```python
from build123d import *

# Parameters (mm, degrees)
SALIENTE_EXTRUIR1_DEPTH = 15.875
REDONDEO1_R             = 15.875
CORTAR_EXTRUIR1_REACH   = 48.084
CROQUIS2_R              = 9.525
CORTAR_EXTRUIR2_START   = -3.175
CROQUIS3_R              = 12.7
CORTAR_EXTRUIR2_DEPTH   = 43.909243503
CROQUIS4_R              = 3.2639
CROQUIS4_R_2            = 2.4892
CORTAR_EXTRUIR3_DEPTH   = 47.084243503
REDONDEO2_R             = 1.27
REDONDEO3_R             = 2.54


with BuildPart() as part:
    # Croquis1 → Saliente-Extruir1 (new body)
    with BuildSketch(Plane.XY):
        Polygon((30.48, 0), (-30.48, 0), (-30.48, 6.35), (12.046472996, 38.277805334), (30.48, 6.35), align=None)
    extrude(amount=SALIENTE_EXTRUIR1_DEPTH)

    # Redondeo1
    redondeo1_edges = [part.edges().sort_by_distance(p)[0] for p in [
        (12.046472996, 38.277805334, 7.9375),
    ]]
    fillet(redondeo1_edges, radius=REDONDEO1_R)

    # Croquis2 → Cortar-Extruir1 (cut, up to next)
    with BuildSketch(Plane.XY.offset(15.875), mode=Mode.PRIVATE) as cortar_extruir1_sk1:
        with Locations((7.254003, 16.09860686)):
            Circle(CROQUIS2_R)
    cortar_extruir1_tool1 = extrude(cortar_extruir1_sk1.sketch, amount=-CORTAR_EXTRUIR1_REACH, mode=Mode.PRIVATE) & part.part
    add(cortar_extruir1_tool1.solids().sort_by_distance((7.254003, 16.098607, 15.875))[0], mode=Mode.SUBTRACT)

    # Croquis3 → Cortar-Extruir2 (cut, through all)
    with BuildSketch(Plane.XY.offset(15.875).offset(CORTAR_EXTRUIR2_START)):
        with Locations((7.254003, 16.09860686)):
            Circle(CROQUIS3_R)
    extrude(amount=-CORTAR_EXTRUIR2_DEPTH, mode=Mode.SUBTRACT)

    # Croquis4 → Cortar-Extruir3 (cut, through all)
    with BuildSketch(Plane.XZ):
        with Locations((-23.8125, 11.43)):
            Circle(CROQUIS4_R)
        with Locations(Location((23.8125, 11.43, 0), (0, 0, 210.56660833))):
            Circle(CROQUIS4_R)
        with Locations((7.254003, 9.525)):
            Circle(CROQUIS4_R_2)
    extrude(amount=-CORTAR_EXTRUIR3_DEPTH, mode=Mode.SUBTRACT)

    # Redondeo2
    redondeo2_edges = [part.edges().sort_by_distance(p)[0] for p in [
        (30.48, 0, 7.9375),
        (-30.48, 0, 7.9375),
    ]]
    fillet(redondeo2_edges, radius=REDONDEO2_R)

    # Redondeo3
    redondeo3_edges = [part.edges().sort_by_distance(p)[0] for p in [
        (-30.48, 6.35, 7.9375),
        (30.48, 6.35, 7.9375),
    ]]
    fillet(redondeo3_edges, radius=REDONDEO3_R)


solid = part.part
```
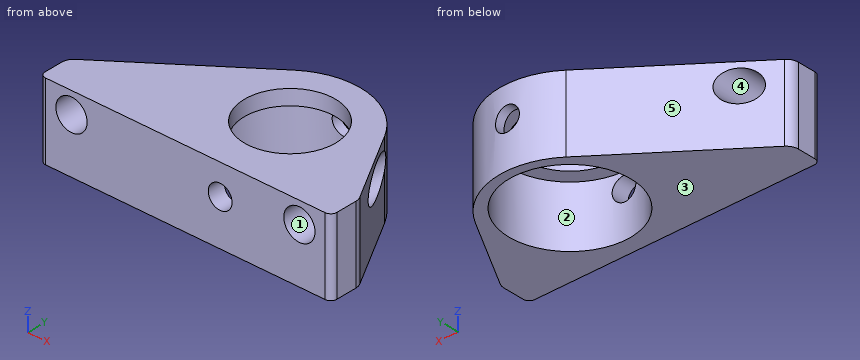
Design review of the part built by this model. Coordinates are the model's own, in mm. Face numbers are marked on the shaded views. A direction names the side the tool comes from. Round coordinates to 2 decimals unless told otherwise and drop trailing zeros. Write each loop counter-clockwise with the first axis right and the second up, starting at its lowest first coordinate (ties: lowest second). Pieces come first, ordered by that corner, then holes. Notation, with made-up numbers: (-15, 41.25) -> (33, 41.25) arc R14 ccw to (33, 60.25) -> close; hole circle Ø5 at (-8.75, 18.25). An arc over 180 degrees is marked (long way). Write item = value, one per line. Start each with the question number.
1) Wall thickness on probe 1 along X at (y, z) = (7.5, 11.43); probe 2 along Z at (x, y) = (23, 3.5) (3 decimals); probe 3 along X at (y, z) = (6.75, 11.43): over which ranges is each line inside the solid? List them lowest first. Write a range as from..to.
2) Take a section at A-A, the plane z = 11.43. State the section outline as (x, y) points (3 decimals).
3) Take a section at B-B, the plane y = 20. State the section outline as (x, z) points (1 decimal), plus the area to 3 significant figures.
4) Mouldability with a two-part tool opening along X and no side actions: class the marked faces 3, 4 and 5 as +X half, -X half, draft (parallel to the pull), parting line (faces both ways), or undercut.
5) Take a section at C-C, the plane x = 8. State the section outline as (y, z) points (3 decimals).
6) Tool access review of the marked faces 1 and 2: name each direction out of +Z, -Z, +X, -X, +Y, -Y from which nothing blocks a thin tool from reaching the whole face with its end or side.
7) Clearance check with flat-ended pins moving along their axes: pin 1 (2 mm diameter, centred on y = 10.5, z = 13.5, fed in from +X); pin 2 (10 mm diameter, centred on x = -1, y = 5, fed in from -Z); pin 3 (8.5 mm diameter, centred on x = -23.81, z = 11.43, fed in from +Y); pin 4 (1.5 mm diameter, centred on y = 11, z = 4.5, fed in from +X). State where each tip first meets the part, or that it passes through.
8) Take a section at D-D, the plane z = 1.75. State the section outline as (x, y) points (3 decimals), plus the area to 3 significant figures.
Results list:
q1.probe_1 = -28.95..-27.08, -20.55..-2.09, 16.6..20.55, 27.08..29.82
q1.probe_2 = 0..8.269, 14.591..15.875
q1.probe_3 = -29.85..-27.08, -20.55..-1.34, 15.85..20.55, 27.08..30.24
q2.outline = (-30.48, 1.27) arc R1.27 ccw to (-29.21, 0) -> (-27.076, 0) -> (-27.076, 8.905) -> (-29.465, 7.112) arc R2.54 ccw to (-30.48, 5.081) -> close; (-20.549, 0) -> (5.652, 0) -> (5.652, 3.5) arc R12.7 cw to (5.652, 28.697) -> (5.652, 30.623) arc R15.875 ccw to (-2.277, 27.524) -> (-20.549, 13.806) -> close; (8.856, 0) -> (20.549, 0) -> (20.549, 23.504) arc R15.875 ccw to (8.856, 30.623) -> (8.856, 28.697) arc R12.7 cw to (8.856, 3.5) -> close; (27.076, 0) -> (29.21, 0) arc R1.27 ccw to (30.48, 1.27) -> (30.48, 5.669) arc R2.54 ccw to (30.14, 6.939) -> (27.076, 12.245) -> close
q3.outline = (-12.3, 0) -> (-4.8, 0) -> (-4.8, 12.7) -> (-1.4, 12.7) -> (-1.4, 15.9) -> (-12.3, 15.9) -> close; (15.9, 12.7) -> (19.3, 12.7) -> (19.3, 0) -> (22.6, 0) -> (22.6, 8.4) arc R3.3 cw to (22.6, 14.5) -> (22.6, 15.9) -> (15.9, 15.9) -> close
q3.area = 183 mm²
q4.face_3 = draft
q4.face_4 = undercut
q4.face_5 = -X half
q5.outline = (0, 0) -> (3.421, 0) -> (3.421, 7.15) -> (0, 7.15) -> close; (0, 11.9) -> (3.421, 11.9) -> (3.421, 12.7) -> (6.603, 12.7) -> (6.603, 15.875) -> (0, 15.875) -> close; (25.594, 12.7) -> (28.777, 12.7) -> (28.777, 11.9) -> (30.686, 11.9) -> (30.686, 15.875) -> (25.594, 15.875) -> close; (28.777, 0) -> (30.686, 0) -> (30.686, 7.15) -> (28.777, 7.15) -> close
q6.face_1 = +Y, -Y
q6.face_2 = -Z
q7.pin_1 = 28.66
q7.pin_2 = 0
q7.pin_3 = 14.55
q7.pin_4 = 28.23
q8.outline = (-30.48, 1.27) arc R1.27 ccw to (-29.21, 0) -> (29.21, 0) arc R1.27 ccw to (30.48, 1.27) -> (30.48, 5.669) arc R2.54 ccw to (30.14, 6.939) -> (21.002, 22.766) arc R15.875 ccw to (-2.277, 27.524) -> (-29.465, 7.112) arc R2.54 ccw to (-30.48, 5.081) -> close; hole circle Ø25.4 at (7.254, 16.099)
q8.area = 781 mm²
